Part model, mm, in its own coordinate system. Give positions to 0.01 mm unless a question says otherwise; leave off trailing zeros. Order: outer loops, then holes, each group sorted by start corner. A loop starts at its lowest first (then second) coordinate and runs counter-clockwise, first axis right, second up.
1. Slice it at A-A on x = 0.75. List the corners of the cut face in (y, z), and give its area (3 significant figures).
2. Drop flat-ended pins along their axis: pin 1 Ø2 at (x, z) = (0, 65) entering from +Y; pin 2 Ø0.6 at (x, y) = (0, 2) entering from +Z; pin 3 Ø1 at (x, z) = (1.5, 29) entering from -Y. Give the stop position or say it passes through.
3. Probe line 1 (Z direction, x = -0.65, y = 1.85); line 2 (X direction, y = 0.05, z = 64). List the from-to ranges inside material, lowest first.
4. Slice it at B-B on z = 20.5. List the corners of the cut face in (x, y).
Autodesk Fusion 360 part; units mm, degrees
sketch "Sketch1" plane through (0, 0, 0) normal (0, 0, 1) x (1, 0, 0)
  circle A0 centre (0, 0) radius 2.35
  dimension "d1" = 4.7
extrude "Extrude1" add sketch "Sketch1" along normal blind 4.2
sketch "Sketch2" plane through (0, 0, 4.2) normal (0, 0, 1) x (-1, 0, 0)
  circle A0 centre (0, 0) radius 2.35
  circle A1 centre (0, 0) radius 1.6
  dimension "d4" = 3.2
extrude "Extrude2" add sketch "Sketch2" along normal blind 100 from surface at -4.2 contours A1
sketch "Sketch3" plane through (0, 0, 4.2) normal (0, 0, 1) x (-1, 0, 0)
  circle A0 centre (0, 0) radius 1.6
  circle A1 centre (0, 0) radius 2.35
  line L0 (1.7212, -1.6) -> (-1.7212, -1.6)
  line L1 (1.7212, 1.6) -> (-1.7212, 1.6)
extrude "Extrude3" add sketch "Sketch3" along normal blind 0.2 contours A0 A1 L0 L1 | A0 A1 L0 L1
sketch "Sketch4" plane through (0, 0, 4.4) normal (0, 0, 1) x (-1, 0, 0)
  arc A0 (1.7212, -1.6) -> (1.7212, 1.6) centre (0, 0) ccw
  line L0 (1.7212, 1.6) -> (0, 1.6)
  arc A1 (0, -1.6) -> (0, 1.6) centre (0, 0) ccw
  line L1 (0, -1.6) -> (1.7212, -1.6)
  line L2 (0, 1.6) -> (-1.7212, 1.6)
  arc A2 (-1.7212, 1.6) -> (-1.7212, -1.6) centre (0, 0) ccw
  line L3 (-1.7212, -1.6) -> (0, -1.6)
  arc A3 (0, 1.6) -> (0, -1.6) centre (0, 0) ccw
  line L4 (1.6, -1.6) -> (1.6, 1.6)
  line L5 (-1.6, 1.6) -> (-1.6, -1.6)
extrude "Extrude4" add sketch "Sketch4" along normal blind 0.2 contours A1 L1 L4 | L0 A1 L4 | L3 A3 L5 | L2 A3 L5
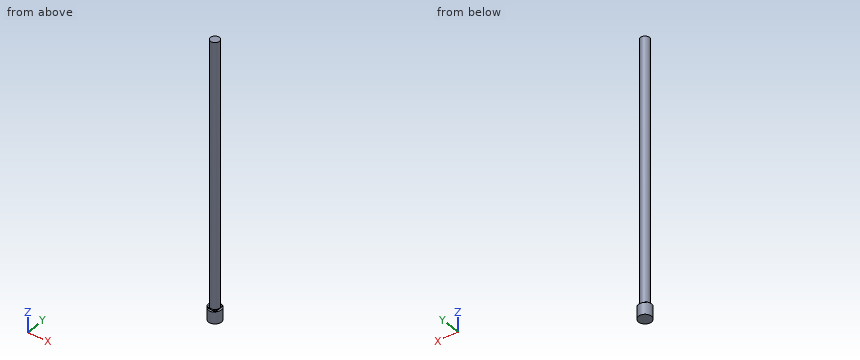
Data:
1. outline: (-2.23, 0) - (2.23, 0) - (2.23, 4.2) - (1.6, 4.2) - (1.6, 4.6) - (1.41, 4.6) - (1.41, 100) - (-1.41, 100) - (-1.41, 4.6) - (-1.6, 4.6) - (-1.6, 4.2) - (-2.23, 4.2) - close
1. area: 290 mm2
2. pin 1: stops at y = 1.6
2. pin 2: stops at z = 4.2
2. pin 3: stops at y = -1.25
3. line 1: z = 0 to 4.2
3. line 2: x = -1.6 to 1.6
4. outline: circle Ø3.2 at (0, 0)
